The model under review builds one solid part; all positions refer to its coordinate system, in mm. Face numbers are marked on the shaded views. A direction names the side the tool comes from. Coordinates: 2 decimals unless noted, no trailing zeros. Order: outer loops, then holes, each group sorted by start corner. A loop starts at its lowest first (then second) coordinate and runs counter-clockwise, first axis right, second up. Notation, with made-up numbers: (43, 64) -> (49, 64) arc R32 ccw to (49, 97) -> close; hole circle Ø9 at (41.5, -33.75). An arc over 180 degrees is marked (long way). Use one line per item in the form item = value.
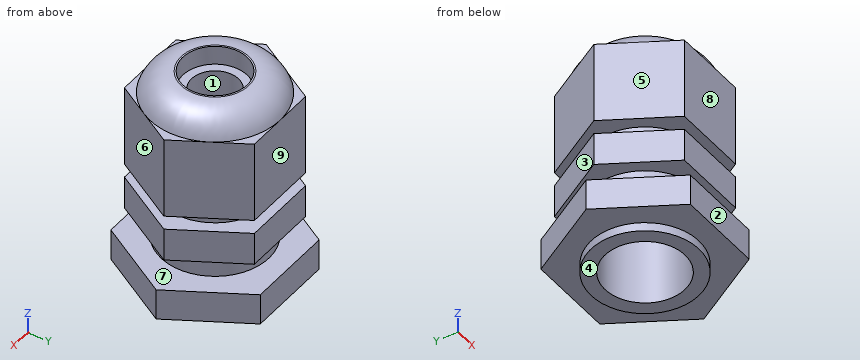
from build123d import *

# Parameters (mm, degrees)
BOSS_EXTRUDE1_DEPTH = 11.75
SKETCH2_R           = 7.75
BOSS_EXTRUDE2_DEPTH = 2
BOSS_EXTRUDE3_DEPTH = 4.75
SKETCH4_R           = 7.75
BOSS_EXTRUDE4_DEPTH = 3.5
BOSS_EXTRUDE5_DEPTH = 4.5
SKETCH6_R           = 7.75
BOSS_EXTRUDE6_DEPTH = 1.25
SKETCH7_R           = 5.75
CUT_EXTRUDE1_DEPTH  = 20
SKETCH8_R           = 9.35
BOSS_EXTRUDE7_DEPTH = 3.25
SKETCH9_R           = 4.625
CUT_EXTRUDE2_DEPTH  = 2.75
FILLET2_R           = 4.725
SKETCH10_R          = 3.375
CUT_EXTRUDE3_DEPTH  = 33.675806544


with BuildPart() as part:
    # Sketch1 → Boss-Extrude1 (new body)
    with BuildSketch(Plane.XY):
        Polygon((10.796450034, 0), (5.398225017, 9.35), (-5.398225017, 9.35), (-10.796450034, 0), (-5.398225017, -9.35), (5.398225017, -9.35), align=None)
    extrude(amount=BOSS_EXTRUDE1_DEPTH)

    # Sketch2 → Boss-Extrude2 (add)
    with BuildSketch(Plane(origin=(0, 0, 0), x_dir=(-1, 0, 0), z_dir=(0, 0, -1))):
        Circle(SKETCH2_R)
    extrude(amount=BOSS_EXTRUDE2_DEPTH)

    # Sketch3 → Boss-Extrude3 (add)
    with BuildSketch(Plane(origin=(0, 0, -2), x_dir=(-1, 0, 0), z_dir=(0, 0, -1))):
        Polygon((10.796450034, 0), (5.398225017, 9.35), (-5.398225017, 9.35), (-10.796450034, 0), (-5.398225017, -9.35), (5.398225017, -9.35), align=None)
    extrude(amount=BOSS_EXTRUDE3_DEPTH)

    # Sketch4 → Boss-Extrude4 (add)
    with BuildSketch(Plane(origin=(0, 0, -6.75), x_dir=(-1, 0, 0), z_dir=(0, 0, -1))):
        Circle(SKETCH4_R)
    extrude(amount=BOSS_EXTRUDE4_DEPTH)

    # Sketch5 → Boss-Extrude5 (add)
    with BuildSketch(Plane(origin=(0, 0, -10.25), x_dir=(-1, 0, 0), z_dir=(0, 0, -1))):
        Polygon((12.413030788, 0), (6.206515394, 10.75), (-6.206515394, 10.75), (-12.413030788, 0), (-6.206515394, -10.75), (6.206515394, -10.75), align=None)
    extrude(amount=BOSS_EXTRUDE5_DEPTH)

    # Sketch6 → Boss-Extrude6 (add)
    with BuildSketch(Plane(origin=(0, 0, -14.75), x_dir=(-1, 0, 0), z_dir=(0, 0, -1))):
        Circle(SKETCH6_R)
    extrude(amount=BOSS_EXTRUDE6_DEPTH)

    # Sketch7 → Cut-Extrude1 (cut)
    with BuildSketch(Plane(origin=(0, 0, -16), x_dir=(-1, 0, 0), z_dir=(0, 0, -1))):
        Circle(SKETCH7_R)
    extrude(amount=-CUT_EXTRUDE1_DEPTH, mode=Mode.SUBTRACT)

    # Sketch8 → Boss-Extrude7 (add)
    with BuildSketch(Plane.XY.offset(11.75)):
        with Locations(Location((0, 0, 0), (0, 0, 210))):
            Circle(SKETCH8_R)
    extrude(amount=BOSS_EXTRUDE7_DEPTH)

    # Sketch9 → Cut-Extrude2 (cut)
    with BuildSketch(Plane.XY.offset(15)):
        Circle(SKETCH9_R)
    extrude(amount=-CUT_EXTRUDE2_DEPTH, mode=Mode.SUBTRACT)

    # Fillet2
    # the kernel refuses this fillet: 4.725 mm, written as the material it takes off along each edge
    with BuildSketch(Plane(origin=(0, 0, 15), x_dir=(-0.8660254037844385, -0.5000000000000001, 0), z_dir=(-0.5000000000000001, 0.8660254037844385, 0))) as fillet2_piece_1:
        with BuildLine():
            CenterArc((4.861124863, -4.725), FILLET2_R, 18.190012051, 71.809987949)
            Line((4.861124863, 0), (4.861124863, 0.0945))
            Line((4.861124863, 0.0945), (9.35, 0.0945))
            Line((9.35, 0.0945), (9.4445, 0))
            ThreePointArc((9.4445, 0), (9.4445, -1.625), (9.439777503, -3.2205))
            Line((9.439777503, -3.2205), (9.35, -3.25))
        make_face()
    revolve(axis=Axis((0, 0, 15), (0, 0, 1)), mode=Mode.SUBTRACT)

    # Sketch10 → Cut-Extrude3 (cut, through all)
    with BuildSketch(Plane.XY.offset(12.25)):
        Circle(SKETCH10_R)
    extrude(amount=-CUT_EXTRUDE3_DEPTH, mode=Mode.SUBTRACT)


solid = part.part
Item 1: Draft analysis for pull direction Y (two halves, no side actions). For the marked faces 1, 2, 3 and 4, state which applies: released by +Y, released by -Y, zero draft, split by the parting line, or undercut.
Results found:
face_1 = undercut
face_2 = released by -Y
face_3 = released by +Y
face_4 = zero draft
Item 2: We need section A-A (z = -14). Write out the cut boundary in (x, y).
Results found:
outline = (-12.41, 0) -> (-6.21, -10.75) -> (6.21, -10.75) -> (12.41, 0) -> (6.21, 10.75) -> (-6.21, 10.75) -> close; hole circle Ø11.5 at (0, 0)
Item 3: To check wall thickness, follow L1, parallel to Y at x = 0, z = -8.5; L2, parallel to Y at x = 0, z = 7 (3 decimals); L3, parallel to Z at x = -5.75, y = 7.25. State the ranges of each line that lie inside material, in increasing order. Write a range as from..to.
Results found:
L1 = -7.75..-5.75, 5.75..7.75
L2 = -9.35..-3.375, 3.375..9.35
L3 = -14.75..-10.25, -6.75..-2, 0..12.02
Item 4: We need section C-C (y = -8.5). State how many separate pieces and enclosed holes the cut face has, plus the area to 3 significant figures.
Results found:
separate_pieces = 3
enclosed_holes = 0
area = 270 mm²
Item 5: We need section B-B (z = 1). Write out the cut boundary in (x, y), plus the area to 3 significant figures.
Results found:
outline = (-10.8, 0) -> (-5.4, -9.35) -> (5.4, -9.35) -> (10.8, 0) -> (5.4, 9.35) -> (-5.4, 9.35) -> close; hole circle Ø11.5 at (0, 0)
area = 199 mm²
Item 6: Clearance check with flat-ended pins moving along their axes: pin 1 (4 mm diameter, centred on x = -4.5, z = 1.5, fed in from +Y); pin 2 (1.5 mm diameter, centred on x = 0.5, y = 7.5, fed in from +Z); pin 3 (6 mm diameter, centred on x = 7, z = 4, fed in from -Y); pin 4 (1 mm diameter, centred on x = -1, y = 0.5, fed in from +Z). State where each tip first meets the part, or that it passes through.
Results found:
pin_1 = 9.35
pin_2 = 14.6
pin_3 = -9.35
pin_4 = through
Item 7: Tool access review of the marked faces 5, 6, 7, 8 and 9: name each direction out of +Z, -Z, +X, -X, +Y, -Y from which nothing blocks a thin tool from reaching the whole face with its end or side.
Results found:
face_5 = +Z, -X, -Y
face_6 = +Z, +X, -Y
face_7 = none
face_8 = +Z, +X, -X, -Y
face_9 = +Z, +X, -X, +Y
